from build123d import *

# Parameters (mm, degrees)
F1_DEPTH = 6
F3_DEPTH = 6
F4_W     = 25
F4_H     = 12
F5_DEPTH = 6
F6_D     = 13


with BuildPart() as f1:
    # F0 (on Front) → F1 (new body)
    with BuildSketch(Plane.XZ):
        with BuildLine():
            Line((32, 6.5), (32, 12.5))
            Line((32, 12.5), (-32, 12.5))
            Line((-32, 12.5), (-32, -12.5))
            Line((-32, -12.5), (32, -12.5))
            Line((32, -12.5), (32, -6.5))
            Line((32, -6.5), (12, -6.5))
            ThreePointArc((12, -6.5), (5.5, 0), (12, 6.5))
            Line((12, 6.5), (32, 6.5))
        make_face()
    extrude(amount=F1_DEPTH)

    # F2 (on face) → F3 (join)
    with BuildSketch(Plane(origin=(-32, 0, 0), x_dir=(0, -1, 0), z_dir=(-1, 0, 0))):
        with BuildLine():
            Line((18, 12.5), (0, 12.5))
            Line((0, 12.5), (0, -12.5))
            Line((0, -12.5), (18, -12.5))
            ThreePointArc((18, -12.5), (5.5, 0), (18, 12.5))
        make_face()
        with BuildLine():
            ThreePointArc((30.5, 0), (26.8388347648, 8.8388347648), (18, 12.5))
            Line((18, 12.5), (18, 6.5))
            ThreePointArc((18, 6.5), (22.5961940777, 4.5961940777), (24.5, 0))
            ThreePointArc((24.5, 0), (22.5961940777, -4.5961940777), (18, -6.5))
            Line((18, -6.5), (18, -12.5))
            ThreePointArc((18, -12.5), (26.8388347648, -8.8388347648), (30.5, 0))
        make_face()
        with BuildLine():
            Line((18, 6.5), (18, 12.5))
            ThreePointArc((18, 12.5), (5.5, 0), (18, -12.5))
            Line((18, -12.5), (18, -6.5))
            ThreePointArc((18, -6.5), (11.5, 0), (18, 6.5))
        make_face()
    extrude(amount=F3_DEPTH)

    # F4 (on face) → F5 (join)
    with BuildSketch(Plane.XY.offset(12.5)):
        with BuildLine():
            ThreePointArc((-13, 12), (-25.5, 24.5), (-38, 12))
            Line((-38, 12), (-13, 12))
        make_face()
        Polygon((-38, 0), (-38, -6), (-32, -6), (-13, -6), (-13, 0), align=None)
        with Locations((-25.5, 6)):
            Rectangle(F4_W, F4_H)
    extrude(amount=-F5_DEPTH)

    # F6 (through all)
    with Locations(Plane.XY.offset(12.5)):
        with Locations((-25.5, 12)):
            Hole(F6_D / 2)


solid = f1.part
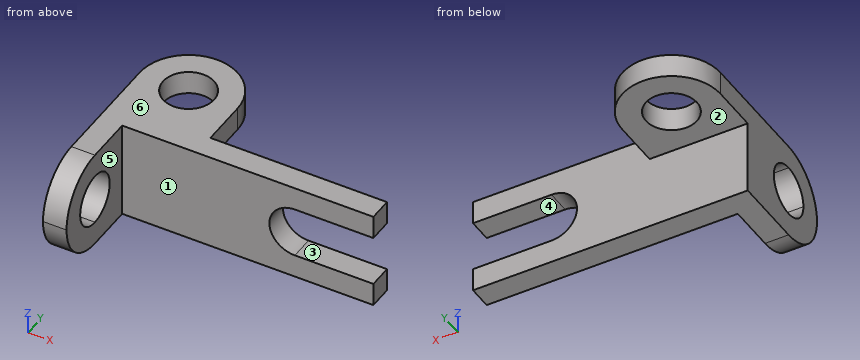
Here's how the part is built. I have some questions about the finished solid (model axes, mm). Face numbers are marked on the shaded views. A direction names the side the tool comes from. Round coordinates to 2 decimals unless told otherwise and drop trailing zeros. Write each loop counter-clockwise with the first axis right and the second up, starting at its lowest first coordinate (ties: lowest second). Pieces come first, ordered by that corner, then holes. Notation, with made-up numbers: (52, 35.5) -> (109, 35.5) arc R35 ccw to (109, 67.5) -> close; hole circle Ø9 at (85.25, 23.25). An arc over 180 degrees is marked (long way). One line per item, written item: value.
1) Suppose I cut it at C-C on y = -1. List the corners of the cut face in (x, z) for me.
Filled sheet:
outline: (-38, -12.5) -> (32, -12.5) -> (32, -6.5) -> (12, -6.5) arc R6.5 cw to (12, 6.5) -> (32, 6.5) -> (32, 12.5) -> (-38, 12.5) -> close
2) Suppose I cut it at A-A on y = 9.5. List the corners of the cut face in (x, z) for me.
Filled sheet:
outline: (-38, 6.5) -> (-31.5, 6.5) -> (-31.5, 12.5) -> (-38, 12.5) -> close; (-19.5, 6.5) -> (-13, 6.5) -> (-13, 12.5) -> (-19.5, 12.5) -> close
3) We'd pull the mould along Z, two halves only. Please class the marked faces 1, 2 and 3: released by +Z, released by -Z, zero draft, split by the parting line, or undercut.
Filled sheet:
face 1: zero draft
face 2: released by -Z
face 3: undercut
4) I'm going to push flat-ended pins straight in: pin 1 Ø12 at (x, z) = (-19.5, 0.5) entering from -Y; pin 2 Ø4 at (x, z) = (-14.5, 4) entering from +Y; pin 3 Ø5 at (y, z) = (6, 10) entering from +X. Where does each tip first touch, or does it pass through?
Filled sheet:
pin 1: stops at y = -6
pin 2: stops at y = 0
pin 3: stops at x = -13
5) If I drill on line 1 (Y direction, x = -25.5, z = 11.1); line 2 (Z direction, x = -18.5, y = 13.5); line 3 (Y direction, x = 24, z = -10.75), over which ranges is the centre line in solid material (lowest first)? Write a range as [from, to].
Filled sheet:
line 1: y = [-6, 5.5], [18.5, 24.5]
line 2: z = [6.5, 12.5]
line 3: y = [-6, 0]
6) For the marked faces 4, 5 and 6, which set-ups out of +Z, -Z, +X, -X, +Y, -Y let a thin tool reach every point of the face, with its end or its side?
Filled sheet:
face 4: +X, +Y, -Y
face 5: +Z, -Z, +X, -Y
face 6: +Z, +X, -X, +Y, -Y
7) Suppose I cut it at B-B on x = -25.5. List the corners of the cut face in (y, z) for me.
Filled sheet:
outline: (-6, -12.5) -> (0, -12.5) -> (0, 6.5) -> (5.5, 6.5) -> (5.5, 12.5) -> (-6, 12.5) -> close; (18.5, 6.5) -> (24.5, 6.5) -> (24.5, 12.5) -> (18.5, 12.5) -> close
8) Suppose I cut it at D-D on z = 3.5. List the corners of the cut face in (x, y) for me.
Filled sheet:
outline: (-38, -30) -> (-32, -30) -> (-32, -23.48) -> (-38, -23.48) -> close; (-38, -12.52) -> (-32, -12.52) -> (-32, -6) -> (6.52, -6) -> (6.52, 0) -> (-38, 0) -> close
